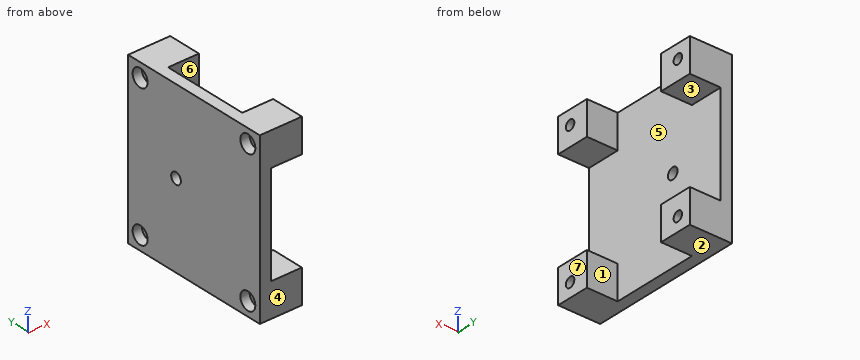
```python
from build123d import *

# Parameters (mm, degrees)
SKETCH1_W                                      = 76.2
SKETCH1_H                                      = 69.85
BOSS_EXTRUDE1_DEPTH                            = 19.05
CUT_EXTRUDE1_DEPTH                             = 13.97
CBORE_FOR_8_SOCKET_HEAD_CAP_SCREW1_D           = 4.4958
CBORE_FOR_8_SOCKET_HEAD_CAP_SCREW1_CBORE_D     = 7.9375
CBORE_FOR_8_SOCKET_HEAD_CAP_SCREW1_CBORE_DEPTH = 4.1656
F_1_4_20_TAPPED_HOLE1_D                        = 5.1054
F_1_4_20_TAPPED_HOLE1_DEPTH                    = 19.05
F_1_4_20_TAPPED_HOLE1_TIP                      = 1.533816902


with BuildPart() as part:
    # Sketch1 → Boss-Extrude1 (new body)
    with BuildSketch(Plane(origin=(0, 0, 0), x_dir=(0, 0, -1), z_dir=(1, 0, 0))):
        Rectangle(SKETCH1_W, SKETCH1_H)
    extrude(amount=BOSS_EXTRUDE1_DEPTH)

    # Sketch2 → Cut-Extrude1 (cut)
    with BuildSketch(Plane(origin=(19.05, 0, 0), x_dir=(0, 0, -1), z_dir=(1, 0, 0))):
        Polygon((-22.86, -34.925), (22.86, -34.925), (22.86, -19.685), (38.1, -19.685), (38.1, 19.685), (22.86, 19.685), (22.86, 34.925), (-22.86, 34.925), (-22.86, 19.685), (-38.1, 19.685), (-38.1, -19.685), (-22.86, -19.685), align=None)
    extrude(amount=-CUT_EXTRUDE1_DEPTH, mode=Mode.SUBTRACT)

    # CBORE for #8 Socket Head Cap Screw1 (through all)
    with Locations(Plane(origin=(0, -5.74842533, -9.122205943), x_dir=(0, 0, -1), z_dir=(-1, 0, 0))):
        with Locations((-40.872205943, -34.32342533), (22.627794057, -34.32342533), (22.627794057, 22.82657467), (-40.872205943, 22.82657467)):
            CounterBoreHole(CBORE_FOR_8_SOCKET_HEAD_CAP_SCREW1_D / 2, CBORE_FOR_8_SOCKET_HEAD_CAP_SCREW1_CBORE_D / 2, CBORE_FOR_8_SOCKET_HEAD_CAP_SCREW1_CBORE_DEPTH)

    # 1/4-20 Tapped Hole1
    with Locations(Plane(origin=(5.08, 0, 0), x_dir=(0, 0, -1), z_dir=(1, 0, 0))):
        with Locations((0, 9.525)):
            Hole(F_1_4_20_TAPPED_HOLE1_D / 2, depth=F_1_4_20_TAPPED_HOLE1_DEPTH)
            with Locations((0, 0, -(F_1_4_20_TAPPED_HOLE1_DEPTH + F_1_4_20_TAPPED_HOLE1_TIP / 2))):  # 118° drill point
                Cone(0, F_1_4_20_TAPPED_HOLE1_D / 2, F_1_4_20_TAPPED_HOLE1_TIP, mode=Mode.SUBTRACT)


solid = part.part
```
The listing builds one solid part. Answer for the finished solid, in the listing's coordinates (mm). Face numbers are marked on the shaded views. A direction names the side the tool comes from. Coordinates: 2 decimals unless noted, no trailing zeros. Write each loop counter-clockwise with the first axis right and the second up, starting at its lowest first coordinate (ties: lowest second). Pieces come first, ordered by that corner, then holes. Notation, with made-up numbers: (69.25, 65.25) - (104.25, 65.25) arc R18 ccw to (104.25, 92.25) - close; hole circle Ø11 at (30.25, -15.75). An arc over 180 degrees is marked (long way). Return JSON: item names as keys, results as strings. Group by question number.
Q1. The part is cut by section D-D on z = -13.5. Write down the section's boundary in (x, y) (3 decimals).
Q2. Flat-ended cylindrical pins translate along their axes: pin 1 Ø1 at (y, z) = (-9, -21.5) entering from -X; pin 2 Ø5 at (y, z) = (28.575, 31.75) entering from -X; pin 3 Ø4 at (y, z) = (-28.575, 31.75) entering from -X; pin 4 Ø2 at (y, z) = (-4, 0.5) entering from +X. Find the tip coordinate at first contact, or state that the pin passes through.
Q3. The part is cut by section C-C on z = 0. Write down the section's boundary in (x, y) (3 decimals).
Q4. Find the intervals of material crossed by line 1 along Z through (x, y) = (15.5, 28.5); line 2 along Y through (x, z) = (8.75, -31.75) (3 decimals); line 3 along Y through (x, z) = (2.4, -31.75) (3 decimals), in increasing order. Write a range as [from, to].
Q5. The part is cut by section B-B on x = 12. Write down the section's boundary in (y, z) (3 decimals).
Q6. For a pull along Y with two mould halves and no side action, classify the marked faces 4, 5, 6 and 7 as +Y half, -Y half, draft (parallel to the pull), parting line (faces both ways), or undercut.
Q7. Which of the six approach directions +Z, -Z, +X, -X, +Y, -Y give full straight-line access (tool end or side, diameter ignored) to the marked faces 1, 2 and 3?
Q8. The part is cut by section A-A on z = -31.75. Write down the section's boundary in (x, y) (3 decimals), and give its area (3 significant figures).
Evaluation:
{
 "1": {"outline": "(0, -34.925) - (5.08, -34.925) - (5.08, 34.925) - (0, 34.925) - close"},
 "2": {"pin 1": "stops at x = 0", "pin 2": "stops at x = 4.17", "pin 3": "passes through", "pin 4": "stops at x = 5.08"},
 "3": {"outline": "(0, -34.925) - (5.08, -34.925) - (5.08, 6.972) - (0, 6.972) - close; (0, 12.078) - (5.08, 12.078) - (5.08, 34.925) - (0, 34.925) - close"},
 "4": {"line 1": "z = [-38.1, -34], [-29.5, -22.86], [22.86, 29.5], [34, 38.1]", "line 2": "y = [-34.925, -30.823], [-26.327, -19.685], [19.685, 26.327], [30.823, 34.925]", "line 3": "y = [-34.925, -32.544], [-24.606, 24.606], [32.544, 34.925]"},
 "5": {"outline": "(-34.925, -38.1) - (-19.685, -38.1) - (-19.685, -22.86) - (-34.925, -22.86) - close; (-34.925, 22.86) - (-19.685, 22.86) - (-19.685, 38.1) - (-34.925, 38.1) - close; (19.685, -38.1) - (34.925, -38.1) - (34.925, -22.86) - (19.685, -22.86) - close; (19.685, 22.86) - (34.925, 22.86) - (34.925, 38.1) - (19.685, 38.1) - close; hole circle Ø4.496 at (-28.575, -31.75); hole circle Ø4.496 at (-28.575, 31.75); hole circle Ø4.496 at (28.575, -31.75); hole circle Ø4.496 at (28.575, 31.75)"},
 "6": {"face 4": "-Y half", "face 5": "undercut", "face 6": "undercut", "face 7": "draft"},
 "7": {"face 1": "+Z, -Z, +X", "face 2": "-Z, +X, -X, +Y, -Y", "face 3": "+X, +Y, -Y"},
 "8": {"outline": "(0, -34.925) - (19.05, -34.925) - (19.05, -30.823) - (4.166, -30.823) - (4.166, -32.544) - (0, -32.544) - close; (0, -24.606) - (4.166, -24.606) - (4.166, -26.327) - (19.05, -26.327) - (19.05, -19.685) - (5.08, -19.685) - (5.08, 19.685) - (19.05, 19.685) - (19.05, 26.327) - (4.166, 26.327) - (4.166, 24.606) - (0, 24.606) - close; (0, 32.544) - (4.166, 32.544) - (4.166, 30.823) - (19.05, 30.823) - (19.05, 34.925) - (0, 34.925) - close", "area": "581 mm2"}
}
